For this review, take the finished solid that the model builds, in its own axes (mm). Face numbers are marked on the shaded views. A direction names the side the tool comes from. Give positions to 0.01 mm unless a question says otherwise; leave off trailing zeros. Order: outer loops, then holes, each group sorted by start corner. A loop starts at its lowest first (then second) coordinate and runs counter-clockwise, first axis right, second up. Notation, with made-up numbers: (86.25, 65.5) - (144.25, 65.5) arc R28 cw to (144.25, 83.5) - close; hole circle Ø10 at (-15.5, 22). An arc over 180 degrees is marked (long way). Answer as a JSON object with one key per item and string values. Group by question number.
from build123d import *

# Parameters (mm, degrees)
BOSS_EXTRUDE1_DEPTH                 = 200
SKETCH4_R                           = 10
BOSS_EXTRUDE4_DEPTH                 = 40
BOSS_EXTRUDE5_START                 = 100
SKETCH5_R                           = 10
BOSS_EXTRUDE5_DEPTH                 = 100
CUT_EXTRUDE1_REACH                  = 302.47
CUT_EXTRUDE1_END_RADIUS             = 10
SKETCH6_W                           = 5
SKETCH6_H                           = 15
CUT_EXTRUDE1_DIRECTION_2_REACH      = 302.47
CUT_EXTRUDE1_DIRECTION_2_END_RADIUS = 10


with BuildPart() as part:
    # Sketch1 → Boss-Extrude1 (new body)
    with BuildSketch(Plane(origin=(0, 0, 0), x_dir=(1, 0, 0), z_dir=(0, 1, 0))):
        Polygon((12.701705922, 0), (6.350852961, 11), (-6.350852961, 11), (-12.701705922, 0), (-6.350852961, -11), (6.350852961, -11), align=None)
    extrude(amount=BOSS_EXTRUDE1_DEPTH)

    # Sketch4 → Boss-Extrude4 (add)
    with BuildSketch(Plane.XZ):
        with Locations(Location((0, 0, 0), (0, 0, 90))):
            Circle(SKETCH4_R)
    extrude(amount=BOSS_EXTRUDE4_DEPTH)

    # Sketch5 → Boss-Extrude5 (add)
    with BuildSketch(Plane(origin=(0, 200, 0), x_dir=(1, 0, 0), z_dir=(0, 1, 0)).offset(BOSS_EXTRUDE5_START)):
        with Locations(Location((0, 0, 0), (0, 0, 270))):
            Circle(SKETCH5_R)
    extrude(amount=-BOSS_EXTRUDE5_DEPTH)

    # Cut-Extrude1: up to this cylinder (the profile starts inside it)
    cut_extrude1_end = Plane(origin=(0, 247.5, 0), z_dir=(0, -1, 0)) * Cylinder(CUT_EXTRUDE1_END_RADIUS, 625.94, mode=Mode.PRIVATE)
    # Sketch6 → Cut-Extrude1 (cut, up to the surface)
    with BuildSketch(Plane.XY, mode=Mode.PRIVATE) as cut_extrude1_sk1:
        with Locations((7.5, 247.5)):
            Rectangle(SKETCH6_W, SKETCH6_H)
    cut_extrude1_tool1 = extrude(cut_extrude1_sk1.sketch, amount=-CUT_EXTRUDE1_REACH, mode=Mode.PRIVATE) & cut_extrude1_end
    add(cut_extrude1_tool1.solids().sort_by_distance((7.5, 247.5, 0))[0], mode=Mode.SUBTRACT)

    # Cut-Extrude1 direction 2: up to this cylinder (the profile starts inside it)
    cut_extrude1_direction_2_end = Plane(origin=(0, 247.5, 0), z_dir=(0, -1, 0)) * Cylinder(CUT_EXTRUDE1_DIRECTION_2_END_RADIUS, 625.94, mode=Mode.PRIVATE)
    # Sketch6 → Cut-Extrude1 direction 2 (cut, up to the surface)
    with BuildSketch(Plane.XY, mode=Mode.PRIVATE) as cut_extrude1_direction_2_sk1:
        with Locations((7.5, 247.5)):
            Rectangle(SKETCH6_W, SKETCH6_H)
    cut_extrude1_direction_2_tool1 = extrude(cut_extrude1_direction_2_sk1.sketch, amount=CUT_EXTRUDE1_DIRECTION_2_REACH, mode=Mode.PRIVATE) & cut_extrude1_direction_2_end
    add(cut_extrude1_direction_2_tool1.solids().sort_by_distance((7.5, 247.5, 0))[0], mode=Mode.SUBTRACT)


solid = part.part
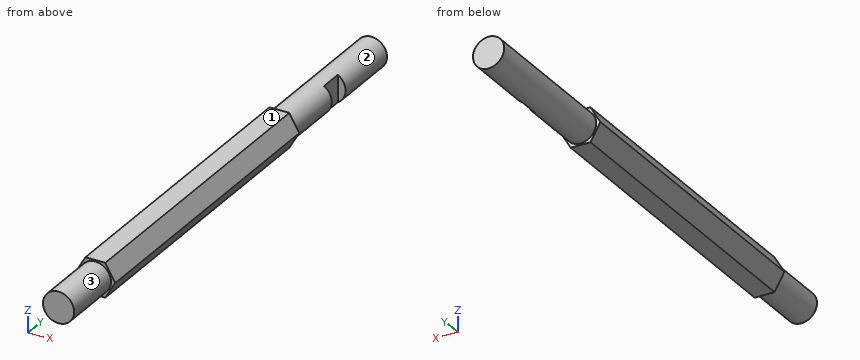
1) Consider section B-B (y = 141). Give the boundary of the cut face in (x, z).
2) Consider section A-A (x = 0). Give the boundary of the cut face in (y, z).
3) Consider section C-C (z = 5.5). Give the boundary of the cut face in (x, y).
4) For the marked faces 1, 2 and 3, list the 3-axis set-ups (+Z, -Z, +X, -X, +Y, -Y) from which the entire face can be reached by the end or side of a thin tool; tool diameter is ignored.
5) For line 1 (Y direction, x = 5.75, z = 7); line 2 (Y direction, x = 7.5, z = 7.5); line 3 (X direction, y = 147, z = 9), list the stretches that pass through material, from the lowest coordinate up.
6) For pin 1 (10 mm diameter, centred on y = 265.5, z = -2.5, fed in from +X); pin 2 (1 mm diameter, centred on y = 18.5, z = -1.5, fed in from +X); pin 3 (12 mm diameter, centred on y = 27, z = 0.5, fed in from +X), all flat-tipped, find the tip position at first contact; note any pin that passes through.
Result set:
{
 "1": {"outline": "(-12.7, 0) - (-6.35, -11) - (6.35, -11) - (12.7, 0) - (6.35, 11) - (-6.35, 11) - close"},
 "2": {"outline": "(-40, -10) - (0, -10) - (0, -11) - (200, -11) - (200, -10) - (300, -10) - (300, 10) - (200, 10) - (200, 11) - (0, 11) - (0, 10) - (-40, 10) - close"},
 "3": {"outline": "(-9.53, 0) - (-8.35, 0) - (-8.35, -40) - (8.35, -40) - (8.35, 0) - (9.53, 0) - (9.53, 200) - (8.35, 200) - (8.35, 240) - (5, 240) - (5, 255) - (8.35, 255) - (8.35, 300) - (-8.35, 300) - (-8.35, 200) - (-9.53, 200) - close"},
 "4": {"face 1": "+Z, +X, -X, +Y, -Y", "face 2": "+Y", "face 3": "-Y"},
 "5": {"line 1": "y = -40 to 240, 255 to 300", "line 2": "y = 0 to 200", "line 3": "x = -7.51 to 7.51"},
 "6": {"pin 1": "stops at x = 10", "pin 2": "stops at x = 12.12", "pin 3": "stops at x = 12.7"}
}
